Read the model definition and answer for the solid it produces. Units are mm, in the model's axes. A direction names the side the tool comes from. Give positions to 0.01 mm unless a question says otherwise; leave off trailing zeros. Order: outer loops, then holes, each group sorted by start corner. A loop starts at its lowest first (then second) coordinate and runs counter-clockwise, first axis right, second up. Notation, with made-up numbers: (-18.75, 35) - (20.25, 35) arc R9 ccw to (20.25, 39) - close; hole circle Ø9 at (-0.5, 0). An arc over 180 degrees is marked (long way). Return JSON: item names as keys, results as strings.
Autodesk Inventor part; units mm, degrees
ref_plane "YZ Plane" through (0, 0, 0) normal (1, 0, 0) x (0, 1, 0)
ref_plane "XZ Plane" through (0, 0, 0) normal (0, 1, 0) x (-1, 0, 0)
ref_plane "XY Plane" through (0, 0, 0) normal (0, 0, 1) x (1, 0, 0)
sketch "Sketch1" plane through (0, 0, 0) normal (0, 1, 0) x (-1, 0, 0)
  line L0 (-22.05, -28.75) -> (22.05, -28.75)
  line L1 (22.05, -28.75) -> (22.05, 28.75)
  line L2 (22.05, 28.75) -> (-22.05, 28.75)
  line L3 (-22.05, 28.75) -> (-22.05, -28.75)
  line L4 (-22.05, -28.75) -> (22.05, 28.75) construction
  line L5 (22.05, -28.75) -> (-22.05, 28.75) construction
  point P0 (0, 0)
  dimension "d0" = 57.5
  dimension "d1" = 44.1
extrude "Extrusion1" add sketch "Sketch1" along normal blind 1.5
chamfer "Chamfer1" distance 2 angle 45 1 edges at (-22.05, 0.75, -28.75)
sketch "Sketch4" plane through (0, 1.5, 0) normal (0, 1, 0) x (1, 0, 0)
  line L0 (22.6381, -25.9185) -> (13.7388, -25.9185)
  line L1 (13.7388, -25.9185) -> (13.7388, -21.956)
  line L2 (13.7388, -21.956) -> (22.6381, -21.956)
  line L3 (22.6381, -21.956) -> (22.6381, -25.9185)
  line L4 (11.4165, -21.956) -> (0.7633, -21.956)
  line L5 (0.7633, -21.956) -> (0.7633, -24.4569)
  line L6 (0.7633, -24.4569) -> (11.4165, -24.4569)
  line L7 (11.4165, -24.4569) -> (11.4165, -21.956)
  line L8 (-0.6658, -26.6006) -> (-6.707, -26.6006)
  line L9 (-6.707, -26.6006) -> (-6.707, -22.3783)
  line L10 (-6.707, -22.3783) -> (-0.6658, -22.3783)
  line L11 (-0.6658, -22.3783) -> (-0.6658, -26.6006)
  line L12 (-6.707, -24.392) -> (-14.5426, -24.392)
  line L13 (-14.5426, -24.392) -> (-14.5426, -21.0953)
  line L14 (-14.5426, -21.0953) -> (-6.707, -21.0953)
  line L15 (-6.707, -21.0953) -> (-6.707, -24.392)
  line L16 (-14.5426, -21.0953) -> (-11.8996, -21.0953)
  line L17 (-11.8996, -21.0953) -> (-11.8996, -19.5363)
  line L18 (-11.8996, -19.5363) -> (-14.5426, -19.5363)
  line L19 (-14.5426, -19.5363) -> (-14.5426, -21.0953)
  line L20 (-21.1238, -24.2621) -> (-17.4211, -24.2621)
  line L21 (-17.4211, -24.2621) -> (-17.4211, -21.956)
  line L22 (-17.4211, -21.956) -> (-21.1238, -21.956)
  line L23 (-21.1238, -21.956) -> (-21.1238, -24.2621)
  line L24 (5.6616, -20.7705) -> (1.894, -20.7705)
  line L25 (1.894, -20.7705) -> (1.894, -17.3277)
  line L26 (1.894, -17.3277) -> (5.6616, -17.3277)
  line L27 (5.6616, -17.3277) -> (5.6616, -20.7705)
  line L28 (-2.848, -19.9261) -> (-5.2515, -19.9261)
  line L29 (-5.2515, -19.9261) -> (-5.2515, -18.3346)
  line L30 (-5.2515, -18.3346) -> (-2.848, -18.3346)
  line L31 (-2.848, -18.3346) -> (-2.848, -19.9261)
  line L32 (-17.2689, -17.0029) -> (-14.5426, -17.0029)
  line L33 (-14.5426, -17.0029) -> (-14.5426, -13.4952)
  line L34 (-14.5426, -13.4952) -> (-17.2689, -13.4952)
  line L35 (-17.2689, -13.4952) -> (-17.2689, -17.0029)
  line L36 (15.925, -11.4814) -> (12.4173, -11.4814)
  line L37 (12.4173, -11.4814) -> (12.4173, -14.7294)
  line L38 (12.4173, -14.7294) -> (15.925, -14.7294)
  line L39 (15.925, -14.7294) -> (15.925, -11.4814)
  line L40 (-2.1335, 9.0455) -> (1.894, 9.0455)
  line L41 (1.894, 9.0455) -> (1.894, -8.9481)
  line L42 (1.894, -8.9481) -> (-2.1335, -8.9481)
  line L43 (-2.1335, -8.9481) -> (-2.1335, 9.0455)
  line L44 (4.5573, 3.3291) -> (1.6991, 3.3291)
  line L45 (1.6991, 3.3291) -> (1.6991, 0.6009)
  line L46 (1.6991, 0.6009) -> (4.5573, 0.6009)
  line L47 (4.5573, 0.6009) -> (4.5573, 3.3291)
  line L48 (-17.5287, 13.7631) -> (-14.1519, 13.7631)
  line L49 (-14.1519, 13.7631) -> (-14.1519, 10.4096)
  line L50 (-14.1519, 10.4096) -> (-17.5287, 10.4096)
  line L51 (-17.5287, 10.4096) -> (-17.5287, 13.7631)
  line L52 (16.8052, 16.3739) -> (14.7212, 16.3739)
  line L53 (14.7212, 16.3739) -> (14.7212, 12.4259)
  line L54 (14.7212, 12.4259) -> (16.8052, 12.4259)
  line L55 (16.8052, 12.4259) -> (16.8052, 16.3739)
  line L56 (-23.3919, 26.0219) -> (-13.2211, 26.0219)
  line L57 (-13.2211, 26.0219) -> (-13.2211, 21.0711)
  line L58 (-13.2211, 21.0711) -> (-23.3919, 21.0711)
  line L59 (-23.3919, 21.0711) -> (-23.3919, 26.0219)
  line L60 (-20.3793, 16.7032) -> (-17.8455, 16.7032)
  line L61 (-17.8455, 16.7032) -> (-17.8455, 19.4346)
  line L62 (-17.8455, 19.4346) -> (-20.3793, 19.4346)
  line L63 (-20.3793, 19.4346) -> (-20.3793, 16.7032)
  line L64 (-11.5832, 21.8169) -> (-0.7032, 21.8169)
  line L65 (-0.7032, 21.8169) -> (-0.7032, 24.5446)
  line L66 (-0.7032, 24.5446) -> (-11.5832, 24.5446)
  line L67 (-11.5832, 24.5446) -> (-11.5832, 21.8169)
  line L68 (-2.5673, 18.6812) -> (-4.8458, 18.6812)
  line L69 (-4.8458, 18.6812) -> (-4.8458, 22.2038)
  line L70 (-4.8458, 22.2038) -> (-2.5673, 22.2038)
  line L71 (-2.5673, 22.2038) -> (-2.5673, 18.6812)
  line L72 (0.9146, 27.1153) -> (6.539, 27.1153)
  line L73 (6.539, 27.1153) -> (6.539, 22.2038)
  line L74 (6.539, 22.2038) -> (0.9146, 22.2038)
  line L75 (0.9146, 22.2038) -> (0.9146, 27.1153)
  line L76 (2.2307, 17.9158) -> (4.5573, 17.9158)
  line L77 (4.5573, 17.9158) -> (4.5573, 22.2038)
  line L78 (4.5573, 22.2038) -> (2.2307, 22.2038)
  line L79 (2.2307, 22.2038) -> (2.2307, 17.9158)
  line L80 (6.0899, 24.1958) -> (14.5454, 24.1958)
  line L81 (14.5454, 24.1958) -> (14.5454, 21.5323)
  line L82 (14.5454, 21.5323) -> (6.0899, 21.5323)
  line L83 (6.0899, 21.5323) -> (6.0899, 24.1958)
  line L84 (14.2886, 21.5323) -> (11.9019, 21.5323)
  line L85 (11.9019, 21.5323) -> (11.9019, 19.3557)
  line L86 (11.9019, 19.3557) -> (14.2886, 19.3557)
  line L87 (14.2886, 19.3557) -> (14.2886, 21.5323)
  line L88 (21.4363, 24.0758) -> (17.64, 24.0758)
  line L89 (17.64, 24.0758) -> (17.64, 21.5323)
  line L90 (17.64, 21.5323) -> (21.4363, 21.5323)
  line L91 (21.4363, 21.5323) -> (21.4363, 24.0758)
  point P0 (0, 0)
  point P1 (6.539, 24.1958)
  point P2 (6.0899, 22.2038)
extrude "Clearance Cutouts" cut sketch "Sketch4" against normal blind 1.5
sketch "Sketch5" plane through (0, 1.5, 0) normal (0, 1, 0) x (1, 0, 0)
  line L0 (9.9457, 22.5156) -> (-6.9835, 22.5156) construction
  line L1 (9.9457, 17.9158) -> (-6.9835, 17.9158)
  line L2 (-6.9835, 27.1153) -> (9.9457, 27.1153)
  arc A0 (9.9457, 17.9158) -> (9.9457, 27.1153) centre (9.9457, 22.5156) ccw
  arc A1 (-6.9835, 27.1153) -> (-6.9835, 17.9158) centre (-6.9835, 22.5156) ccw
  line L3 (-11.5832, 24.5446) -> (-0.7032, 24.5446)
  line L4 (0.9146, 22.2038) -> (0.9146, 27.1153)
  line L5 (-13.2211, 26.0219) -> (-13.2211, 21.0711)
  line L6 (-11.5832, 21.8169) -> (-11.5832, 24.5446)
  line L7 (14.5454, 24.1958) -> (14.5454, 21.5323)
  line L8 (-10.0926, -22.1506) -> (6.9665, -22.1506) construction
  line L9 (-10.0926, -26.6006) -> (6.9665, -26.6006)
  line L10 (6.9665, -17.7006) -> (-10.0926, -17.7006)
  arc A2 (-10.0926, -17.7006) -> (-10.0926, -26.6006) centre (-10.0926, -22.1506) ccw
  arc A3 (6.9665, -26.6006) -> (6.9665, -17.7006) centre (6.9665, -22.1506) ccw
  point P0 (0, 0)
  point P1 (1.4811, 22.5156)
  point P2 (14.5454, 22.5156)
  point P3 (-11.5832, 22.5156)
  point P4 (4.5573, 17.9158)
  point P5 (-1.5631, -22.1506)
  point P6 (-0.6658, -26.6006)
  point P7 (11.4165, -22.1506)
  point P8 (11.4165, -24.4569)
  point P9 (-14.5426, -22.1506)
  point P10 (-14.5426, -19.5363)
  dimension "d53" = 8.9
extrude "Extrusion4" cut sketch "Sketch5" against normal blind 1.5 contours L1 A1 L2 A0 | A2 L10 A3 L9
sketch "Sketch6" plane through (0, 0, 0) normal (0, -1, 0) x (1, 0, 0)
  line L0 (22.05, 21.956) -> (22.05, -28.75)
  line L1 (22.05, -16.5) -> (-12.45, -16.5)
  line L2 (-12.45, -16.5) -> (-12.45, 16.5)
  line L3 (-12.45, 16.5) -> (22.05, 16.5)
  line L4 (22.05, 16.5) -> (22.05, -16.5)
  point P0 (0, 0)
  point P1 (22.05, 16.5)
  dimension "d44" = 33
  dimension "d45" = 34.5
  dimension "d46" = 16.5
extrude "Extrusion5" cut sketch "Sketch6" against normal through all
sketch "Sketch7" plane through (0, 1.5, 0) normal (0, 1, 0) x (1, 0, 0)
  line L0 (-22.05, -28.75) -> (22.05, -28.75)
  arc A0 (4, -28.75) -> (-4, -28.75) centre (0, -28.75) ccw
  line L1 (22.05, 28.75) -> (-20.05, 28.75)
  arc A1 (-4, 28.75) -> (4, 28.75) centre (0, 28.75) ccw
  line L2 (22.05, 28.75) -> (-20.05, 28.75)
  point P0 (0, 0)
  point P1 (4, 28.75)
  dimension "d49" = 4
  dimension "d50" = 4
extrude "Extrusion6" add sketch "Sketch7" against normal up to surface (1.5 mm away)
equation "\"d50\" = d49"
properties part number "Flex Holder V1" material "Thermoplastic Resin"
Q1. A cutting plane is placed at D-D (y = 1). Give the number of separate pieces and of enclosed holes in the cut face, and give its area (3 significant figures).
Values:
{"separate pieces": "1", "enclosed holes": "7", "area": "853 mm²"}
Q2. Given pin 1 (0.8 mm diameter, centred on y = 1, z = 23, fed in from +X); pin 2 (5 mm diameter, centred on x = 0.5, z = -21, fed in from +Y); pin 3 (12 mm diameter, centred on x = 10.5, z = 12, fed in from +Y), each flat-ended and moving along its own axis, determine where each tip first touches the part or whether it passes through.
Values:
{"pin 1": "stops at x = 13.74", "pin 2": "passes through", "pin 3": "stops at y = 1.5"}
Q3. Consider L1, parallel to X at y = 1.15, z = 23.5; L2, parallel to Z at x = 16.5, y = 0.6; L3, parallel to Z at x = -6.5, y = 1.2. Determine where each line is inside the solid, lowest interval first.
Values:
{"L1": "x = -22.05 to -21.12, -17.42 to -14.54, 11.42 to 13.74", "L2": "z = -28.75 to -16.5, 16.5 to 21.96, 25.92 to 28.75", "L3": "z = -28.75 to -27.12, -17.92 to -16.5, 16.5 to 17.7, 26.6 to 28.75"}
Q4. For faces 1 (the flat face through (-7, 1, 26.601)), 2 (the flat face through (-18, 1, -21.071)), determine the directions among +Z, -Z, +X, -X, +Y, -Y from which every point of the face is accessible in a straight line to the end or side of a thin tool.
Values:
{"face 1": "+Y, -Y", "face 2": "-X, +Y, -Y"}
Q5. Determine the mould class of faces 3 (the flat face through (-21.124, 1, 23)), 4 (the flat face through (0, 1, 28.75)), 5 (the flat face through (22.05, 1, 27)) for opening direction Z: released by +Z, released by -Z, zero draft, split by the parting line, or undercut.
Values:
{"face 3": "undercut", "face 4": "released by +Z", "face 5": "zero draft"}
Q6. A cutting plane is placed at A-A (x = -5.5). Write down the section's boundary in (y, z).
Values:
{"outline": "(0, -28.75) - (1.5, -28.75) - (1.5, -27.12) - (0, -27.12) - close; (0, -17.92) - (1.5, -17.92) - (1.5, -16.5) - (0, -16.5) - close; (0, 16.5) - (1.5, 16.5) - (1.5, 17.7) - (0, 17.7) - close; (0, 26.6) - (1.5, 26.6) - (1.5, 28.75) - (0, 28.75) - close"}
Q7. A cutting plane is placed at C-C (x = 12). Write down the section's boundary in (y, z).
Values:
{"outline": "(0, -28.75) - (1.5, -28.75) - (1.5, -26.63) - (0, -26.63) - close; (0, -18.4) - (1.5, -18.4) - (1.5, -16.5) - (0, -16.5) - close; (0, 16.5) - (1.5, 16.5) - (1.5, 28.75) - (0, 28.75) - close"}
Q8. A cutting plane is placed at B-B (z = 23). Write down the section's boundary in (x, y), and give its area (3 significant figures).
Values:
{"outline": "(-22.05, 0) - (-21.12, 0) - (-21.12, 1.5) - (-22.05, 1.5) - close; (-17.42, 0) - (-14.54, 0) - (-14.54, 1.5) - (-17.42, 1.5) - close; (11.42, 0) - (13.74, 0) - (13.74, 1.5) - (11.42, 1.5) - close", "area": "9.19 mm²"}
